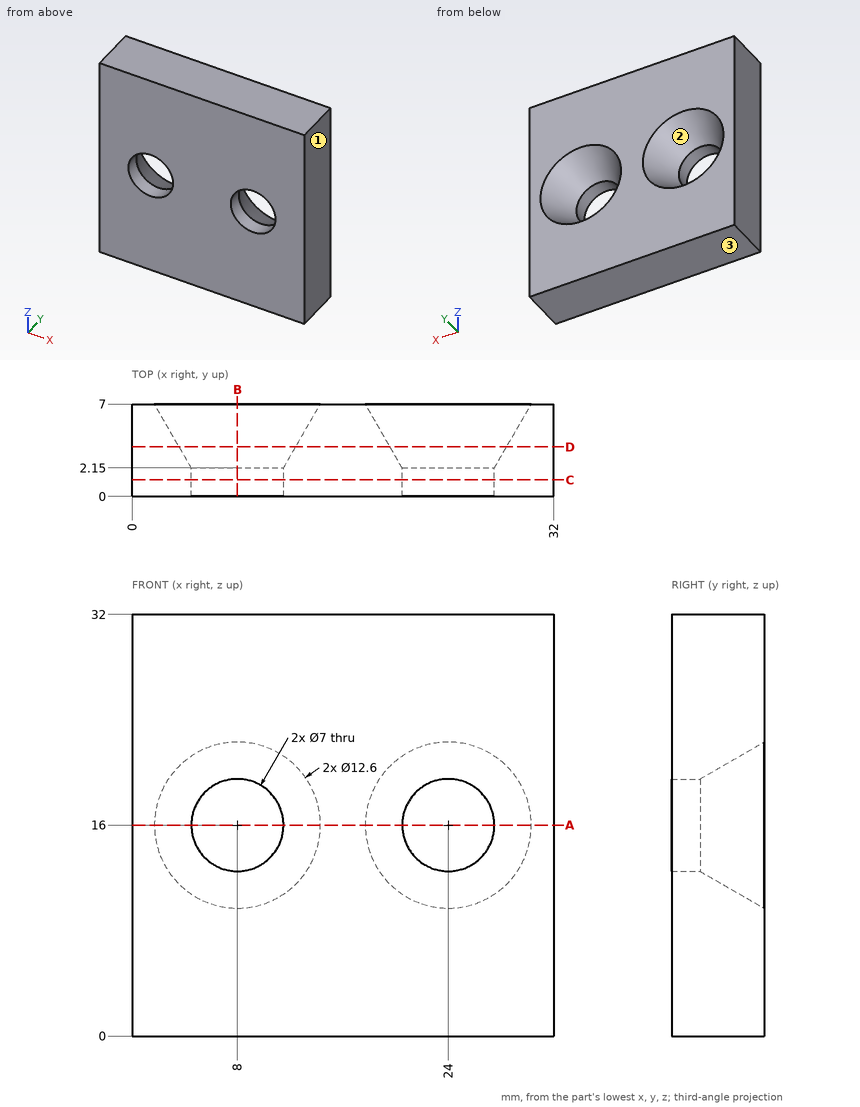
Here's the drawing with two shaded views (mm, measured from the low corner). I have some questions. Give positions to 0.01 mm unless a question says otherwise; leave off trailing zeros. Write each loop counter-clockwise with the first axis right and the second up, starting at its lowest first coordinate (ties: lowest second). Pieces come first, ordered by that corner, then holes. Notation, with made-up numbers: (-10, 13.5) - (3, 13.5) arc R24 cw to (3, 52.5) - close; hole circle Ø4 at (17.5, -6). An arc over 180 degrees is marked (long way). Write item = value, one per line. Start each with the question number.
1. Imagine slicing it at A-A (z = 16). Please give me the cut outline in (x, y).
2. Imagine slicing it at C-C (y = 1.25). Please give me the cut outline in (x, z), and give its area (3 significant figures).
3. Imagine slicing it at B-B (x = 8). Please give me the cut outline in (y, z), and give its area (3 significant figures).
4. Please list where these lines run through material, in increasing order: line 1 (X direction, y = 1, z = 16); line 2 (Z direction, x = 24, y = 1.7); line 3 (X direction, y = 0.5, z = 19) (1 decimal).
5. Imagine slicing it at D-D (y = 3.75). Please give me the cut outline in (x, z), and give its area (3 significant figures).
6. For pin 1 (6.5 mm diameter, centred on x = 24, z = 16, fed in from +Y), with a flat end and sliding along its axis, tell me the tip position at first contact or that it passes through.
7. Thinking about a two-plate mould opening in X: for the marked faces 1, 2 and 3, which applies, released by +X, released by -X, zero draft, split by the parting line, or undercut?
Worked answers:
q1.outline = (0, 0) - (4.5, 0) - (4.5, 2.15) - (1.7, 7) - (0, 7) - close; (11.5, 0) - (20.5, 0) - (20.5, 2.15) - (17.7, 7) - (14.3, 7) - (11.5, 2.15) - close; (27.5, 0) - (32, 0) - (32, 7) - (30.3, 7) - (27.5, 2.15) - close
q2.outline = (0, 0) - (32, 0) - (32, 32) - (0, 32) - close; hole circle Ø7 at (8, 16); hole circle Ø7 at (24, 16)
q2.area = 947 mm2
q3.outline = (0, 0) - (7, 0) - (7, 9.7) - (2.15, 12.5) - (0, 12.5) - close; (0, 19.5) - (2.15, 19.5) - (7, 22.3) - (7, 32) - (0, 32) - close
q3.area = 161 mm2
q4.line_1 = 0 to 4.5, 11.5 to 20.5, 27.5 to 32
q4.line_2 = 0 to 12.5, 19.5 to 32
q4.line_3 = 0 to 6.2, 9.8 to 22.2, 25.8 to 32
q5.outline = (0, 0) - (32, 0) - (32, 32) - (0, 32) - close; hole circle Ø8.85 at (8, 16); hole circle Ø8.85 at (24, 16)
q5.area = 901 mm2
q6.pin_1 = through
q7.face_1 = released by +X
q7.face_2 = undercut
q7.face_3 = zero draft
